Work out the finished part from the listing and answer in its coordinate system (mm). Give positions to 0.01 mm unless a question says otherwise; leave off trailing zeros. Loops run counter-clockwise (first coordinate to the right, second up) from the corner with the lowest first, then second, coordinate; pieces in that order, holes last. Notation, with made-up numbers: (-12.75, 66.25) - (13.25, 66.25) arc R20 ccw to (13.25, 74.25) - close; hole circle Ø9 at (-38, 13.5). An arc over 180 degrees is marked (long way). One line per item, written item: value.
from build123d import *

# Parameters (mm, degrees)
CROQUIS1_R              = 5
CROQUIS1_R_2            = 2
SALIENTE_EXTRUIR1_DEPTH = 6.35
REDONDEO1_R             = 6.35
CROQUIS2_R              = 6.35
CORTAR_EXTRUIR1_DEPTH   = 7.35


with BuildPart() as part:
    # Croquis1 → Saliente-Extruir1 (new body)
    with BuildSketch(Plane(origin=(0, 0, 0), x_dir=(1, 0, 0), z_dir=(0, 1, 0))):
        with BuildLine():
            Line((-22.956480566, 15), (-83.666002653, 15))
            ThreePointArc((-83.666002653, 15), (-85, 0), (-83.666002653, -15))
            ThreePointArc((-83.666002653, -15), (-83.151528449, -17.630181979), (-82.554391371, -20.242837383))
            Line((-82.554391371, -20.242837383), (-53.31124161, -15))
            Line((-53.31124161, -15), (-22.956480566, -15))
            ThreePointArc((-22.956480566, -15), (-20.420534839, -15.528361119), (-18.306603323, -17.025518341))
            ThreePointArc((-18.306603323, -17.025518341), (0, -25), (18.306603323, -17.025518341))
            ThreePointArc((18.306603323, -17.025518341), (20.420534839, -15.528361119), (22.956480566, -15))
            Line((22.956480566, -15), (83.666002653, -15))
            ThreePointArc((83.666002653, -15), (85, 0), (83.666002653, 15))
            ThreePointArc((83.666002653, 15), (83.151528449, 17.630181979), (82.554391371, 20.242837383))
            Line((82.554391371, 20.242837383), (53.31124161, 15))
            Line((53.31124161, 15), (22.956480566, 15))
            ThreePointArc((22.956480566, 15), (20.420534839, 15.528361119), (18.306603323, 17.025518341))
            ThreePointArc((18.306603323, 17.025518341), (0, 25), (-18.306603323, 17.025518341))
            ThreePointArc((-18.306603323, 17.025518341), (-20.420534839, 15.528361119), (-22.956480566, 15))
        make_face()
        Circle(CROQUIS1_R, mode=Mode.SUBTRACT)
        with Locations((0, 17)):
            Circle(CROQUIS1_R_2, mode=Mode.SUBTRACT)
        with Locations((14.722431864, 8.5)):
            Circle(CROQUIS1_R_2, mode=Mode.SUBTRACT)
        with Locations((14.722431864, -8.5)):
            Circle(CROQUIS1_R_2, mode=Mode.SUBTRACT)
        with Locations((0, -17)):
            Circle(CROQUIS1_R_2, mode=Mode.SUBTRACT)
        with Locations((-14.722431864, -8.5)):
            Circle(CROQUIS1_R_2, mode=Mode.SUBTRACT)
        with Locations((-14.722431864, 8.5)):
            Circle(CROQUIS1_R_2, mode=Mode.SUBTRACT)
    extrude(amount=SALIENTE_EXTRUIR1_DEPTH)

    # Redondeo1
    redondeo1_edges = [part.edges().sort_by_distance(p)[0] for p in [
        (53.31124161, 3.175, -15),
        (-53.31124161, 3.175, 15),
    ]]
    fillet(redondeo1_edges, radius=REDONDEO1_R)

    # Croquis2 → Cortar-Extruir1 (cut, through all)
    with BuildSketch(Plane(origin=(0, 6.35, 0), x_dir=(1, 0, 0), z_dir=(0, 1, 0))):
        with Locations((-50, 0)):
            Circle(CROQUIS2_R)
        with Locations((50, 0)):
            Circle(CROQUIS2_R)
    extrude(amount=-CORTAR_EXTRUIR1_DEPTH, mode=Mode.SUBTRACT)


solid = part.part
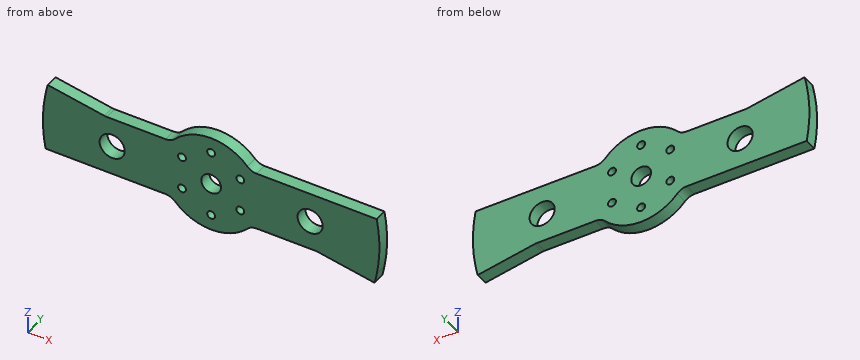
1. Section A-A (x = 0) is taken. Write down the section's boundary in (y, z), and give its area (3 significant figures).
Output:
outline: (0, -25) - (6.35, -25) - (6.35, -19) - (0, -19) - close; (0, -15) - (6.35, -15) - (6.35, -5) - (0, -5) - close; (0, 5) - (6.35, 5) - (6.35, 15) - (0, 15) - close; (0, 19) - (6.35, 19) - (6.35, 25) - (0, 25) - close
area: 203 mm²
2. Find the intervals of material crossed by line 1 along X through (y, z) = (3, 0.5); line 2 along X through (y, z) = (3.5, 8.5); line 3 along Z through (x, y) = (-1.5, 1.5), in increasing order.
Output:
line 1: x = -85 to -56.33, -43.67 to -4.97, 4.97 to 43.67, 56.33 to 85
line 2: x = -84.57 to -16.72, -12.72 to 12.72, 16.72 to 84.57
line 3: z = -24.95 to -18.32, -15.68 to -4.77, 4.77 to 15.68, 18.32 to 24.95
3. Section C-C (z = 8.5) is taken. Write down the section's boundary in (x, y), and give its area (3 significant figures).
Output:
outline: (-84.57, 0) - (-16.72, 0) - (-16.72, 6.35) - (-84.57, 6.35) - close; (-12.72, 0) - (12.72, 0) - (12.72, 6.35) - (-12.72, 6.35) - close; (16.72, 0) - (84.57, 0) - (84.57, 6.35) - (16.72, 6.35) - close
area: 1,020 mm²
4. Section B-B (y = 4.25) is taken. Count the separate pieces of the cut face and the enclosed holes in it, and give its area (3 significant figures).
Output:
separate pieces: 1
enclosed holes: 9
area: 5,390 mm²
5. Flat-ended cylindrical pins translate along their axes: pin 1 Ø1.9 at (x, y) = (48, 3) entering from +Z; pin 2 Ø2 at (x, y) = (-60, 5.5) entering from -Z; pin 3 Ø1.5 at (x, y) = (-65.5, 1) entering from +Z. Find the tip coordinate at first contact, or state that the pin passes through.
Output:
pin 1: stops at z = 15
pin 2: stops at z = -15
pin 3: stops at z = 17.32
6. Section D-D (x = -29) is taken. Write down the section's boundary in (y, z), and give its area (4 significant figures).
Output:
outline: (0, -15) - (6.35, -15) - (6.35, 15) - (0, 15) - close
area: 190.5 mm²
